from build123d import *
from OCP.BRepFilletAPI import BRepFilletAPI_MakeChamfer

# Parameters (mm, degrees)
BOSS_EXTRUDE1_DEPTH = 84.582
BOSS_EXTRUDE2_DEPTH = 3.175
BOSS_EXTRUDE3_DEPTH = 3.175
SKETCH6_W           = 3.175
SKETCH6_H           = 84.582
BOSS_EXTRUDE4_DEPTH = 4.064
SKETCH7_W           = 1.27
SKETCH7_H           = 84.582
BOSS_EXTRUDE5_DEPTH = 2.794
SKETCH8_W           = 0.508
SKETCH8_H           = 78.232
CUT_EXTRUDE1_DEPTH  = 194.545554644
CHAMFER1_SIZE       = 4.88907126
CHAMFER1_SIZE_2     = 3.175
CHAMFER2_SIZE       = 4.88907126
CHAMFER2_SIZE_2     = 3.175
SKETCH11_W          = 3.175
SKETCH11_H          = 56.642
BOSS_EXTRUDE6_DEPTH = 12.7
CHAMFER3_SIZE       = 6.35
SKETCH10_R          = 34.925
SKETCH10_R_2        = 1.651
CUT_EXTRUDE2_DEPTH  = 12.7
CHAMFER4_SIZE       = 3.175
CHAMFER5_SIZE       = 3.175
CHAMFER5_SIZE_2     = 0.850738686
CHAMFER6_SIZE2      = 0.492353937
CHAMFER6_SIZE       = 1.5875
SKETCH12_W          = 13.208
SKETCH12_H          = 2.032
CUT_EXTRUDE3_DEPTH  = 206.621478571
SKETCH13_R          = 38.354
SKETCH13_R_2        = 0.226701536
CUT_EXTRUDE4_DEPTH  = 1.5875
CHAMFER8_SIZE       = 0.604625217
CHAMFER8_SIZE_2     = 3.429
BOSS_EXTRUDE7_DEPTH = 0.762
CHAMFER9_SIZE       = 0.79375
CHAMFER9_SIZE_2     = 0.212684671


# Some blends are built 0.0001 mm under size
with BuildPart() as part:
    # Sketch3 → Boss-Extrude1 (new body)
    with BuildSketch(Plane(origin=(0, 0, 0), x_dir=(1, 0, 0), z_dir=(0, 1, 0))):
        Polygon((0, 0), (57.196097427, 19.065365809), (171.45, 19.065365809), (171.45, 15.890365809), (57.15, 15.890365809), (0, -3.159634191), align=None)
    extrude(amount=BOSS_EXTRUDE1_DEPTH)

    # Sketch4 → Boss-Extrude2 (add)
    with BuildSketch(Plane(origin=(0, 84.582, 0), x_dir=(1, 0, 0), z_dir=(0, 1, 0))):
        Polygon((57.196097427, 19.065365809), (57.196097427, 15.905731618), (0, -3.159634191), (0, 0), align=None)
    extrude(amount=BOSS_EXTRUDE2_DEPTH)

    # Sketch5 → Boss-Extrude3 (add)
    with BuildSketch(Plane(origin=(0, 0, 0), x_dir=(-1, 0, 0), z_dir=(0, -1, 0))):
        Polygon((-57.196097427, 19.065365809), (-57.196097427, 15.905731618), (0, -3.159634191), (0, 0), align=None)
    extrude(amount=BOSS_EXTRUDE3_DEPTH)

    # Sketch6 → Boss-Extrude4 (add)
    with BuildSketch(Plane(origin=(0.947890257, 0, 2.843670772), x_dir=(0.9486832980505139, 0, -0.3162277660168379), z_dir=(0.3162277660168379, 0, 0.9486832980505139))):
        with Locations((4.144335938, 42.291)):
            Rectangle(SKETCH6_W, SKETCH6_H)
    extrude(amount=BOSS_EXTRUDE4_DEPTH)

    # Sketch7 → Boss-Extrude5 (add)
    with BuildSketch(Plane(origin=(2.425627551, 0, -0.808542517), x_dir=(0.31622776601683794, 0, 0.9486832980505139), z_dir=(-0.9486832980505139, 0, 0.31622776601683794))):
        with Locations((6.426492185, 42.291)):
            Rectangle(SKETCH7_W, SKETCH7_H)
    extrude(amount=BOSS_EXTRUDE5_DEPTH)

    # Sketch8 → Cut-Extrude1 (cut, through all)
    with BuildSketch(Plane(origin=(0, 0, 0), x_dir=(-0.9486832980505139, 0, 0.31622776601683794), z_dir=(-0.316227766016838, 0, -0.9486832980505139))):
        with Locations((-47.693985286, 42.291)):
            Rectangle(SKETCH8_W, SKETCH8_H)
        with Locations((-34.84399019, 42.291)):
            Rectangle(SKETCH8_W, SKETCH8_H)
        with Locations((-21.993995095, 42.291)):
            Rectangle(SKETCH8_W, SKETCH8_H)
        with Locations((-9.144, 42.291)):
            Rectangle(SKETCH8_W, SKETCH8_H)
    extrude(amount=-CUT_EXTRUDE1_DEPTH, mode=Mode.SUBTRACT)

    # Chamfer1
    # the kernel refuses this chamfer: 4.88907126, 3.175 mm, written as the material it takes off along each edge
    with BuildSketch(Plane(origin=(45.0055217, 3.175, -15.001840567), x_dir=(-0.955136727602259, 0, 0.2961652099508787), z_dir=(0, 1, 0)), Plane(origin=(32.814945973, 3.175, -10.938315324), x_dir=(-0.955136727602259, 0, 0.29616520995087847), z_dir=(0, 1, 0)), Plane(origin=(20.624370247, 3.175, -6.874790082), x_dir=(-0.9551367276022591, 0, 0.29616520995087875), z_dir=(0, 1, 0)), Plane(origin=(8.43379452, 3.175, -2.81126484), x_dir=(-0.9551367276022591, 0, 0.29616520995087847), z_dir=(0, 1, 0))) as chamfer1_piece_1:
        Polygon((CHAMFER1_SIZE * 0.999777923568, CHAMFER1_SIZE * 0.0210737654668), (-CHAMFER1_SIZE_2 * 0.0210737654663, CHAMFER1_SIZE_2 * 0.999777923546), (0, 0), align=None)
    extrude(amount=78.232, mode=Mode.SUBTRACT)

    # Chamfer2
    # the kernel refuses this chamfer: 4.88907126, 3.175 mm, written as the material it takes off along each edge
    with BuildSketch(Plane(origin=(46.435343073, 3.175, -12.3188135), x_dir=(0.9551367276022592, 0, -0.29616520995087836), z_dir=(0, 1, 0)), Plane(origin=(34.244767346, 3.175, -8.255288258), x_dir=(0.9551367276022591, 0, -0.29616520995087864), z_dir=(0, 1, 0)), Plane(origin=(22.054191619, 3.175, -4.191763015), x_dir=(0.955136727602259, 0, -0.29616520995087864), z_dir=(0, 1, 0)), Plane(origin=(9.863615892, 3.175, -0.128237773), x_dir=(0.955136727602259, 0, -0.29616520995087864), z_dir=(0, 1, 0))) as chamfer2_piece_1:
        Polygon((CHAMFER2_SIZE * 0.999777923568, CHAMFER2_SIZE * 0.0210737654668), (-CHAMFER2_SIZE_2 * 0.0210737654663, CHAMFER2_SIZE_2 * 0.999777923546), (0, 0), align=None)
    extrude(amount=78.232, mode=Mode.SUBTRACT)

    # Sketch11 → Boss-Extrude6 (add)
    with BuildSketch(Plane(origin=(171.45, 0, 0), x_dir=(0, 0, -1), z_dir=(1, 0, 0))):
        with Locations((17.477865809, 42.291)):
            Rectangle(SKETCH11_W, SKETCH11_H)
    extrude(amount=BOSS_EXTRUDE6_DEPTH)

    # Chamfer3
    chamfer3_edges = [part.edges().sort_by_distance(p)[0] for p in [
        (184.15, 13.97, -17.477865809),
        (184.15, 70.612, -17.477865809),
    ]]
    chamfer(chamfer3_edges, length=CHAMFER3_SIZE)

    # Sketch10 → Cut-Extrude2 (cut)
    with BuildSketch(Plane(origin=(0, 0, -19.065365809), x_dir=(-1, 0, 0), z_dir=(0, 0, -1))):
        with Locations((-141.3256, 42.291)):
            Circle(SKETCH10_R)
        with Locations((-161.6456, 80.772)):
            Circle(SKETCH10_R_2)
        with Locations((-121.0056, 80.772)):
            Circle(SKETCH10_R_2)
        with Locations((-121.0056, 3.81)):
            Circle(SKETCH10_R_2)
        with Locations((-161.6456, 3.81)):
            Circle(SKETCH10_R_2)
    extrude(amount=-CUT_EXTRUDE2_DEPTH, mode=Mode.SUBTRACT)

    # Chamfer4
    chamfer4_edges = [part.edges().sort_by_distance(p)[0] for p in [
        (0, 87.757, 1.579817095),
        (0, -3.175, 1.579817095),
    ]]
    chamfer(chamfer4_edges, length=CHAMFER4_SIZE)

    # Chamfer5
    chamfer5_edges_1 = [part.edges().sort_by_distance(p)[0] for p in [
        (114.3, 0, -15.890365809),
    ]]
    chamfer5_side_1 = [part.faces().sort_by_distance(p)[0] for p in [
        (114.3, 0, -15.907380583),
    ]]
    chamfer5_edges_2 = [part.edges().sort_by_distance(p)[0] for p in [
        (114.3, 84.582, -15.890365809),
    ]]
    chamfer5_side_2 = [part.faces().sort_by_distance(p)[0] for p in [
        (114.3, 84.582, -15.907380583),
    ]]
    chamfer5 = BRepFilletAPI_MakeChamfer(part.part.solid().wrapped)
    for e in chamfer5_edges_1:
        chamfer5.Add(CHAMFER5_SIZE - 0.0001, CHAMFER5_SIZE_2 - 0.0001, e.wrapped, chamfer5_side_1[0].wrapped)
    for e in chamfer5_edges_2:
        chamfer5.Add(CHAMFER5_SIZE - 0.0001, CHAMFER5_SIZE_2 - 0.0001, e.wrapped, chamfer5_side_2[0].wrapped)
    add(Compound.cast(chamfer5.Shape()), mode=Mode.REPLACE)  # a hair under: the kernel refuses the full size

    # Chamfer6
    chamfer6_edges = [part.edges().sort_by_distance(p)[0] for p in [
        (57.196097427, 85.746239108, -15.905731618),
    ]]
    chamfer6_side = [part.faces().sort_by_distance(p)[0] for p in [
        (57.196097427, 85.746239108, -15.915578697),
    ]]
    chamfer(chamfer6_edges, length=CHAMFER6_SIZE, length2=CHAMFER6_SIZE2, reference=chamfer6_side[0])

    # Sketch12 → Cut-Extrude3 (cut, through all)
    with BuildSketch(Plane(origin=(0, 0, -19.065365809), x_dir=(-1, 0, 0), z_dir=(0, 0, -1))):
        with Locations((-95.550097427, 80.391)):
            Rectangle(SKETCH12_W, SKETCH12_H)
        with Locations((-95.550097427, 4.191)):
            Rectangle(SKETCH12_W, SKETCH12_H)
    extrude(amount=-CUT_EXTRUDE3_DEPTH, mode=Mode.SUBTRACT)

    # Sketch13 → Cut-Extrude4 (cut)
    with BuildSketch(Plane(origin=(0, 0, -19.065365809), x_dir=(-1, 0, 0), z_dir=(0, 0, -1))):
        with Locations((-141.3256, 42.291)):
            Circle(SKETCH13_R)
        with Locations((-129.898704957, 9.528246972)):
            Circle(SKETCH13_R_2, mode=Mode.SUBTRACT)
    extrude(amount=-CUT_EXTRUDE4_DEPTH, mode=Mode.SUBTRACT)

    # Chamfer8
    # the kernel refuses this chamfer: 3.429, 0.604625217 mm, written as the material it takes off along each edge
    with BuildSketch(Plane(origin=(141.3256, 42.291, -17.477865809), x_dir=(-1, 0, 0), z_dir=(0, -1, 0))) as chamfer8_piece_1_section:
        Polygon((34.925, -CHAMFER8_SIZE), (34.925 + CHAMFER8_SIZE_2, 0), (34.925, 0), align=None)
    chamfer8_piece_1 = revolve(axis=Axis((141.3256, 42.291, -17.477865809), (0, 0, -1)), mode=Mode.PRIVATE)
    chamfer8_piece_1 = chamfer8_piece_1 & Plane(origin=(141.3256, 42.291, -17.229890684), x_dir=(-1, 0, 0), z_dir=(0, 0, -1)) * Cylinder(38.354, 154, mode=Mode.PRIVATE)
    add(chamfer8_piece_1, mode=Mode.SUBTRACT)

    # Sketch14 → Boss-Extrude7 (add)
    with BuildSketch(Plane(origin=(171.45, 0, 0), x_dir=(0, 0, -1), z_dir=(1, 0, 0))):
        Polygon((15.890365809, 70.612), (15.890365809, 83.731261314), (17.477865809, 84.156630657), (17.477865809, 70.612), align=None)
        Polygon((15.890365809, 13.97), (17.477865809, 13.97), (17.477865809, 0.425369343), (15.890365809, 0.850738686), align=None)
    extrude(amount=BOSS_EXTRUDE7_DEPTH)

    # Chamfer9
    chamfer9_edges_1 = [part.edges().sort_by_distance(p)[0] for p in [
        (172.212, 7.197684671, -17.477865809),
    ]]
    chamfer9_side_1 = [part.faces().sort_by_distance(p)[0] for p in [
        (172.212, 7.197684671, -17.473612116),
    ]]
    chamfer9_edges_2 = [part.edges().sort_by_distance(p)[0] for p in [
        (172.212, 7.410369343, -15.890365809),
    ]]
    chamfer9_side_2 = [part.faces().sort_by_distance(p)[0] for p in [
        (172.207746307, 7.410369343, -15.890365809),
    ]]
    chamfer9_edges_3 = [part.edges().sort_by_distance(p)[0] for p in [
        (172.212, 77.384315329, -17.477865809),
    ]]
    chamfer9_side_3 = [part.faces().sort_by_distance(p)[0] for p in [
        (172.207746307, 77.384315329, -17.477865809),
    ]]
    chamfer9_edges_4 = [part.edges().sort_by_distance(p)[0] for p in [
        (172.212, 77.171630657, -15.890365809),
    ]]
    chamfer9_side_4 = [part.faces().sort_by_distance(p)[0] for p in [
        (172.207746307, 77.171630657, -15.890365809),
    ]]
    chamfer9 = BRepFilletAPI_MakeChamfer(part.part.solid().wrapped)
    for e in chamfer9_edges_1:
        chamfer9.Add(CHAMFER9_SIZE - 0.0001, CHAMFER9_SIZE_2 - 0.0001, e.wrapped, chamfer9_side_1[0].wrapped)
    for e in chamfer9_edges_2:
        chamfer9.Add(CHAMFER9_SIZE_2 - 0.0001, CHAMFER9_SIZE - 0.0001, e.wrapped, chamfer9_side_2[0].wrapped)
    for e in chamfer9_edges_3:
        chamfer9.Add(CHAMFER9_SIZE_2 - 0.0001, CHAMFER9_SIZE - 0.0001, e.wrapped, chamfer9_side_3[0].wrapped)
    for e in chamfer9_edges_4:
        chamfer9.Add(CHAMFER9_SIZE_2 - 0.0001, CHAMFER9_SIZE - 0.0001, e.wrapped, chamfer9_side_4[0].wrapped)
    add(Compound.cast(chamfer9.Shape()), mode=Mode.REPLACE)  # a hair under: the kernel refuses the full size


solid = part.part
Work out the finished part from the listing and answer in its coordinate system (mm). A direction names the side the tool comes from. Give positions to 0.01 mm unless a question says otherwise; leave off trailing zeros. Return JSON: item names as keys, results as strings.
Q1. The mould has two halves that part along Y. Classify faces 6 (the face through (0, 43, 2)), 7 (the face through (5, 0, 4)), 8 (the face through (96, 81.407, -18)), 9 (the face through (30, 87.757, -9)): pulls with the +Y half, pulls with the -Y half, needs draft (parallel to the pull), parting line crosses it, or undercut.
Answer below:
{"face 6": "needs draft", "face 7": "pulls with the -Y half", "face 8": "undercut", "face 9": "pulls with the +Y half"}
Q2. Find section A-A, the plane x = 93.5. State how many separate pieces and enclosed holes the cut face has, and give its area (3 significant figures).
Answer below:
{"separate pieces": "3", "enclosed holes": "0", "area": "253 mm^2"}
Q3. Each of these flat-tipped pins is pushed along its axis until it touches: pin 1 (1 mm diameter, centred on x = 93, z = -18, fed in from +Y); pin 2 (6 mm diameter, centred on x = 69, y = 70.5, fed in from +Z); pin 3 (1.6 mm diameter, centred on x = 175, z = -17.5, fed in from -Y). Where does it stop, or does it pass through?
Answer below:
{"pin 1": "stops at y = 84.43", "pin 2": "stops at z = -15.89", "pin 3": "stops at y = 13.97"}
Q4. Which of the six approach directions +Z, -Z, +X, -X, +Y, -Y give full straight-line access (tool end or side, diameter ignored) to faces 1 (the face through (114.91, 0.43, -17.46)), 2 (the face through (9, 3.175, -2)), 3 (the face through (48.447, 41.743, -14.547)), 4 (the face through (105.896, 27.601, -18.283)), 5 (the face through (30, -3.175, -9))?
Answer below:
{"face 1": "+Z, +X, -Y", "face 2": "none", "face 3": "+Z, -X", "face 4": "-Z", "face 5": "+Z, -Z, +X, -X, -Y"}
Q5. Find the intervals of material crossed by line 1 along Z through (x, y) = (84, 42.5); line 2 along Z through (x, y) = (168.5, 16), in increasing order. Write a range as [from, to].
Answer below:
{"line 1": "z = [-19.07, -15.89]", "line 2": "z = [-17.38, -15.89]"}
